Model file for the job. Use its own axes, mm. Face numbers are marked on the shaded views. A direction names the side the tool comes from. Give positions to 0.01 mm unless a question says otherwise; leave off trailing zeros. Write each loop counter-clockwise with the first axis right and the second up, starting at its lowest first coordinate (ties: lowest second). Pieces come first, ordered by that corner, then holes.
```python
from build123d import *

# Parameters (mm, degrees)
F3_DEPTH = 3


with BuildPart() as f1:
    # F0 (on Front) → F1 (revolve)
    with BuildSketch(Plane.XZ):
        Polygon((34.962991, 4), (34.962991, 0), (38.962991, 0), (38.962991, 8), align=None)
        Polygon((4.962991, 3.4), (4.962991, 0), (34.962991, 0), (34.962991, 4), (4.962991, 4), align=None)
        Polygon((1.962991, 3.4), (0, 0), (4.962991, 0), (4.962991, 3.4), align=None)
    revolve(axis=Axis((9.715057, 0, 0), (1, 0, 0)))

    # F2 (on face) → F3 (cut)
    with BuildSketch(Plane.YZ.offset(38.962991)):
        with BuildLine():
            Line((7.858117, 1.5), (-7.858117, 1.5))
            ThreePointArc((-7.858117, 1.5), (-8, 0), (-7.858117, -1.5))
            Line((-7.858117, -1.5), (7.858117, -1.5))
            ThreePointArc((7.858117, -1.5), (7.96445, -0.753348), (8, 0))
            ThreePointArc((8, 0), (7.96445, 0.753348), (7.858117, 1.5))
        make_face()
    extrude(amount=-F3_DEPTH, mode=Mode.SUBTRACT)


solid = f1.part
```
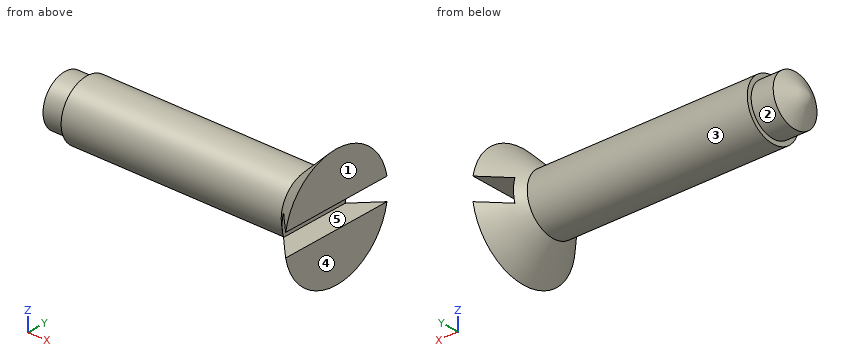
1. Pin check, flat tips, straight feed: P1, Ø2.5, axis at x = 37, y = -2, coming from the -Z side; P2, Ø6, axis at x = 4.5, z = 0, coming from the -Y side; P3, Ø8, axis at x = 21, y = -0.5, coming from the -Z side. Stop position of each tip, or through.
Calculated:
P1: stops at z = -7.05
P2: stops at y = -4
P3: stops at z = -4
2. Pull direction Z, two halves, no side cores. Call the marked faces 3, 4 and 5: +Z half, -Z half, draft (parallel to the pull), parting line (faces both ways), or undercut.
Calculated:
face 3: parting line
face 4: draft
face 5: undercut
3. Which spindle directions (+Z, -Z, +X, -X, +Y, -Y) get a long thin tool onto all of the face, cutting with end or side? Do the marked faces 1 and 2. Say none if no direction does.
Calculated:
face 1: +Z, -Z, +X, +Y, -Y
face 2: -X
4. Slice it at A-A, the plane x = 13. Write the cut outline in (y, z), and give its area (3 significant figures).
Calculated:
outline: circle Ø8 at (0, 0)
area: 50.3 mm2
5. Probe probe 1 along Y at (x, z) = (6, -0.25); probe 2 along Z at (x, y) = (36.5, -0.5); probe 3 along Z at (x, y) = (36, -4). List the from-to ranges inside material, lowest first.
Calculated:
probe 1: y = -3.99 to 3.99
probe 2: z = -5.51 to -1.5, 1.5 to 5.51
probe 3: z = -3.06 to -1.5, 1.5 to 3.06
